from build123d import *

# Parameters (mm, degrees)
BOSS_EXTRUDE1_DEPTH    = 1.651
SKETCH2_W              = 9.525
SKETCH2_H              = 7.62254
CUT_EXTRUDE1_DEPTH     = 18.079855009
BOSS_EXTRUDE2_DEPTH    = 1.524
BOSS_EXTRUDE3_DEPTH    = 1.524
DRAFT1_DEPTH           = 3.175
DRAFT1_2_DEPTH         = 1.651
M2_5_CLEARANCE_HOLE1_D = 2.7051
M3_CLEARANCE_HOLE1_D   = 3.556
FILLET1_R              = 0.23622
FILLET2_R              = 3.429


# Read off the part's stored shape, not the designer's step: Draft1
with BuildPart() as part:
    # Sketch1 → Boss-Extrude1 (new body)
    with BuildSketch(Plane(origin=(0, 1.651, 0), x_dir=(1, 0, 0), z_dir=(0, 1, 0))):
        Polygon((13.490522855, 0), (9.205835634, 10.34415), (-9.205835634, 10.34415), (-13.490522855, 0), (-9.205835634, -10.34415), (13.019017606, -1.138314366), align=None)
    extrude(amount=-BOSS_EXTRUDE1_DEPTH)

    # Sketch2 → Cut-Extrude1 (cut, through all)
    with BuildSketch(Plane.XZ):
        Rectangle(SKETCH2_W, SKETCH2_H)
    extrude(amount=-CUT_EXTRUDE1_DEPTH, mode=Mode.SUBTRACT)

    # Sketch3 → Boss-Extrude2 (add)
    with BuildSketch(Plane(origin=(0, 1.651, 0), x_dir=(-1, 0, 0), z_dir=(0, 1, 0))):
        Polygon((-9.205835634, -10.34415), (-13.490522855, 0), (-13.019017606, 1.138314366), (-4.7625, 4.558275937), (-4.7625, -10.34415), align=None)
    extrude(amount=BOSS_EXTRUDE2_DEPTH)

    # Sketch4 → Boss-Extrude3 (add)
    with BuildSketch(Plane(origin=(0, 1.651, 0), x_dir=(-1, 0, 0), z_dir=(0, 1, 0))):
        Polygon((9.205835634, 10.34415), (13.490522855, 0), (9.205835634, -10.34415), (4.7625, -10.34415), (4.7625, 8.503660118), align=None)
    extrude(amount=BOSS_EXTRUDE3_DEPTH)

    # Draft1 outline → Draft1 (add)
    with BuildSketch(Plane(origin=(0, 0, 0), x_dir=(1, 0, 0), z_dir=(0, 1, 0))):
        Polygon((4.7625, -10.34415), (9.205835634, -10.34415), (13.019017606, -1.138314366), (4.7625, -4.558275937), align=None)
        Polygon((-9.205835634, -10.34415), (-4.7625, -10.34415), (-4.7625, -8.503660118), align=None)
    extrude(amount=DRAFT1_DEPTH)

    # Draft1 2 outline → Draft1 2 (add)
    with BuildSketch(Plane(origin=(0, 0, 0), x_dir=(1, 0, 0), z_dir=(0, 1, 0))):
        Polygon((-4.7625, -10.34415), (4.7625, -10.34415), (4.7625, -4.558275937), (-4.7625, -8.503660118), align=None)
    extrude(amount=DRAFT1_2_DEPTH)

    # M2.5 Clearance Hole1 (through all)
    with Locations(Plane(origin=(0, 3.175, 0), x_dir=(1, 0, 0), z_dir=(0, 1, 0))):
        with Locations((6.914797213, 6.914797213), (-6.914797213, 6.914797213), (-6.914797213, -6.914797213), (6.914797213, -6.914797213)):
            Hole(M2_5_CLEARANCE_HOLE1_D / 2)

    # M3 Clearance Hole1 (through all)
    with Locations(Plane(origin=(0, 3.175, 0), x_dir=(1, 0, 0), z_dir=(0, 1, 0))):
        with Locations((9.779, 0), (-9.779, 0)):
            Hole(M3_CLEARANCE_HOLE1_D / 2)

    # Fillet1
    fillet1_edges = [part.edges().sort_by_distance(p)[0] for p in [
        (4.7625, 0.8255, 3.81127),
        (4.7625, 0.8255, -3.81127),
        (-4.7625, 0.8255, -3.81127),
        (-4.7625, 0.8255, 3.81127),
    ]]
    fillet(fillet1_edges, radius=FILLET1_R)

    # Fillet2
    fillet2_edges = [part.edges().sort_by_distance(p)[0] for p in [
        (9.205835634, 1.5875, 10.34415),
        (-9.205835634, 1.5875, 10.34415),
        (-13.490522855, 1.5875, 0),
        (-9.205835634, 1.5875, -10.34415),
        (9.205835634, 1.5875, -10.34415),
        (13.490522855, 1.5875, 0),
    ]]
    fillet(fillet2_edges, radius=FILLET2_R)


solid = part.part
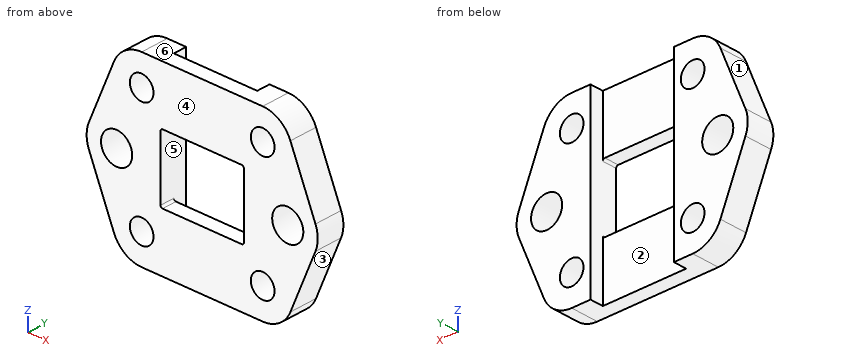
Build history of the part. All positions in model axes, mm. Face numbers are marked on the shaded views. A direction names the side the tool comes from. Coordinates: 2 decimals unless noted, no trailing zeros. Order: outer loops, then holes, each group sorted by start corner. A loop starts at its lowest first (then second) coordinate and runs counter-clockwise, first axis right, second up. Notation, with made-up numbers: (76.25, 68) - (131.25, 68) arc R15 cw to (131.25, 95) - close; hole circle Ø8 at (29, -37.75). An arc over 180 degrees is marked (long way). Put each result on its own line as item: value.
1. Drop flat-ended pins along their axis: P1, Ø2.5, axis at x = 6.91, z = -6.91, coming from the -Y side; P2, Ø1.5, axis at x = 10.5, y = 2, coming from the -Z side; P3, Ø1, axis at y = 1, z = 2.5, coming from the +X side; P4, Ø3.5, axis at x = -1, z = -5.5, coming from the +Y side. Give the stop position or say it passes through.
Answer sheet:
P1: passes through
P2: stops at z = -8.84
P3: stops at x = 12.66
P4: stops at y = 1.65
2. Saw through at A-A (x = 2.75). Write the cut outline in (y, z).
Answer sheet:
outline: (0, -10.34) - (1.65, -10.34) - (1.65, -3.81) - (0, -3.81) - close; (0, 3.81) - (1.65, 3.81) - (1.65, 10.34) - (0, 10.34) - close
3. Probe line 1 along X through (y, z) = (0.4, -1); line 2 along Z through (x, y) = (1.5, 1); line 3 along Z through (x, y) = (-6, 1.3). List the from-to ranges inside material, lowest first. Write a range as [from, to].
Answer sheet:
line 1: x = [-13.06, -11.25], [-8.31, -4.76], [4.76, 8.31], [11.25, 13.06]
line 2: z = [-10.34, -3.81], [3.81, 10.34]
line 3: z = [-10.34, -7.91], [-5.92, 5.92], [7.91, 10.34]
4. Saw through at D-D (x = 10.75). Write the cut outline in (y, z) (3 decimals), and give its area (3 significant figures).
Answer sheet:
outline: (0, -6.616) - (3.175, -6.616) - (3.175, -1.489) - (0, -1.489) - close; (0, 1.489) - (3.175, 1.489) - (3.175, 6.616) - (0, 6.616) - close
area: 32.6 mm^2
5. Tool access for the marked faces 5 and 6: list every direction of +Z, -Z, +X, -X, +Y, -Y with a clear straight run to the whole face (end or side of a thin tool).
Answer sheet:
face 5: +Y
face 6: +Z, +X, -X, +Y, -Y
6. Saw through at B-B (z = 0). Give the number of separate pieces and of enclosed holes in the cut face, and give its area (3 significant figures).
Answer sheet:
separate pieces: 4
enclosed holes: 0
area: 31.0 mm^2
7. Pull direction X, two halves, no side cores. Call the marked faces 1, 2, 3 and 4: pulls with the +X half, pulls with the -X half, needs draft (parallel to the pull), parting line crosses it, or undercut.
Answer sheet:
face 1: pulls with the -X half
face 2: undercut
face 3: pulls with the +X half
face 4: needs draft
